Build history of the part. All positions in model axes, mm. A direction names the side the tool comes from. Give positions to 0.01 mm unless a question says otherwise; leave off trailing zeros. Write each loop counter-clockwise with the first axis right and the second up, starting at its lowest first coordinate (ties: lowest second). Pieces come first, ordered by that corner, then holes. Notation, with made-up numbers: (46.5, 80) -> (59.5, 80) arc R37 cw to (59.5, 116) -> close; hole circle Ø4 at (78, -7). An arc over 180 degrees is marked (long way). Put each result on its own line as item: value.
from build123d import *

# Parameters (mm, degrees)
F0_W     = 45.260496
F0_H     = 48.27787
F1_DEPTH = 25.4
F2_W     = 53.21525
F2_H     = 15.521124
F3_DEPTH = 39.375179
F4_R     = 10.887602
F4_R_2   = 11.039472
F5_DEPTH = 23.324139


with BuildPart() as f1:
    # F0 (on Front) → F1 (new body)
    with BuildSketch(Plane.XZ):
        with Locations((4e-06, -8.146919)):
            Rectangle(F0_W, F0_H)
    extrude(amount=F1_DEPTH)

    # F2 (on Top) → F3 (cut)
    with BuildSketch(Plane.XY):
        with Locations((-0.739105, -22.17301)):
            Rectangle(F2_W, F2_H)
    extrude(amount=-F3_DEPTH, mode=Mode.SUBTRACT)

    # F4 (on Top) → F5 (cut)
    with BuildSketch(Plane.XY):
        with Locations((20.871415, -25.173559)):
            Circle(F4_R)
        with Locations((-24.506071, -24.840043)):
            Circle(F4_R_2)
    extrude(amount=F5_DEPTH, mode=Mode.SUBTRACT)


solid = f1.part
1) Slice it at A-A (x = -2). Write the cut outline in (y, z), plus the area to 3 significant figures.
Filled sheet:
outline: (-25.4, 0) -> (-14.41, 0) -> (-14.41, -32.29) -> (0, -32.29) -> (0, 15.99) -> (-25.4, 15.99) -> close
area: 872 mm2
2) Slice it at D-D (z = -1). Write the cut outline in (x, y).
Filled sheet:
outline: (-22.63, -14.41) -> (22.63, -14.41) -> (22.63, 0) -> (-22.63, 0) -> close
3) Tool access for faces 1 (the flat face through (-22.63, -7, -8)), 2 (the flat face through (0, -14.412, -16)): list every direction of +Z, -Z, +X, -X, +Y, -Y with a clear straight run to the whole face (end or side of a thin tool).
Filled sheet:
face 1: +Z, -Z, -X, +Y, -Y
face 2: -Z, +X, -X, -Y
4) Pin check, flat tips, straight feed: pin 1 (2 mm diameter, centred on x = 16, z = -7.5, fed in from -Y); pin 2 (3 mm diameter, centred on x = 15, z = -1, fed in from -Y); pin 3 (0.5 mm diameter, centred on x = -22, y = -14.5, fed in from +Z). Stop position of each tip, or through.
Filled sheet:
pin 1: y = -14.41
pin 2: y = -16.83
pin 3: z = 0
5) Slice it at B-B (z = 4.5). Write the cut outline in (x, y), plus the area to 3 significant figures.
Filled sheet:
outline: (-22.63, -13.96) arc R11.04 cw to (-13.48, -25.4) -> (9.99, -25.4) arc R10.89 cw to (22.63, -14.43) -> (22.63, 0) -> (-22.63, 0) -> close
area: 954 mm2
6) Wall check: L1, parallel to Y at x = 5.5, z = -1; L2, parallel to Z at x = 0, y = -21.5; L3, parallel to Y at x = -14.5, z = 4.5. Give the ranges that are in metal, low to high.
Filled sheet:
L1: -14.41 to 0
L2: 0 to 15.99
L3: -20.18 to 0
7) Slice it at C-C (y = -21.75). Write the cut outline in (x, z).
Filled sheet:
outline: (-13.91, 0) -> (10.54, 0) -> (10.54, 15.99) -> (-13.91, 15.99) -> close
